Verification items for the finished model (mm, model axes). A direction names the side the tool comes from. Give positions to 0.01 mm unless a question says otherwise; leave off trailing zeros. Write each loop counter-clockwise with the first axis right and the second up, starting at its lowest first coordinate (ties: lowest second). Pieces come first, ordered by that corner, then holes. Notation, with made-up numbers: (-25, 69) - (-4, 69) arc R29 cw to (-4, 103) - close; hole circle Ø8 at (4, -33). An arc over 180 degrees is marked (long way). Put each result on its own line as item: value.
from build123d import *

# Parameters (mm, degrees)
SKETCH1_W           = 32
SKETCH1_H           = 32
SKETCH1_W_2         = 28
SKETCH1_H_2         = 28
BOSS_EXTRUDE1_DEPTH = 20
SKETCH2_W           = 10
SKETCH2_H           = 8
CUT_EXTRUDE1_DEPTH  = 33


with BuildPart() as part:
    # Sketch1 → Boss-Extrude1 (new body)
    with BuildSketch(Plane(origin=(0, 0, 0), x_dir=(1, 0, 0), z_dir=(0, 1, 0))):
        Rectangle(SKETCH1_W, SKETCH1_H)
        Rectangle(SKETCH1_W_2, SKETCH1_H_2, mode=Mode.SUBTRACT)
    extrude(amount=BOSS_EXTRUDE1_DEPTH)

    # Sketch2 → Cut-Extrude1 (cut, through all)
    with BuildSketch(Plane(origin=(16, 0, 0), x_dir=(0, 0, -1), z_dir=(1, 0, 0))):
        with Locations((0, 4)):
            Rectangle(SKETCH2_W, SKETCH2_H)
    extrude(amount=-CUT_EXTRUDE1_DEPTH, mode=Mode.SUBTRACT)


solid = part.part
Q1. Set-up check for faces 5 (the face through (0, 0, 15)), 6 (the face through (-14, 10, 0)), 7 (the face through (-15, 4, 5)): record each of +Z, -Z, +X, -X, +Y, -Y from which the full face is reachable in a straight line by a thin tool's end or side.
Answers follow:
face 5: +Z, -Z, +X, -X, -Y
face 6: +Y, -Y
face 7: +X, -X, -Y
Q2. Scan line: line 1 along Z through (x, y) = (0, 18.75). Record every from-to range of solid material in increasing order.
Answers follow:
line 1: z = -16 to -14, 14 to 16
Q3. Release check for a two-part mould opening along Z. For faces 1 (the face through (0, 10, -16)), 2 (the face through (-15, 4, -5)), 3 (the face through (16, 10, 0)), 4 (the face through (15, 4, 5)) record: released by +Z, released by -Z, zero draft, split by the parting line, or undercut.
Answers follow:
face 1: released by -Z
face 2: undercut
face 3: zero draft
face 4: undercut
Q4. Section check B-B, the plane x = 1. Record the cut outline in (y, z).
Answers follow:
outline: (0, -16) - (20, -16) - (20, -14) - (0, -14) - close; (0, 14) - (20, 14) - (20, 16) - (0, 16) - close
Q5. Section check A-A, the plane z = 3. Record the cut outline in (x, y), plus the area to 3 significant figures.
Answers follow:
outline: (-16, 8) - (-14, 8) - (-14, 20) - (-16, 20) - close; (14, 8) - (16, 8) - (16, 20) - (14, 20) - close
area: 48.0 mm2
Q6. Section check D-D, the plane y = 7.25. Record the cut outline in (x, z), plus the area to 3 significant figures.
Answers follow:
outline: (-16, -16) - (16, -16) - (16, -5) - (14, -5) - (14, -14) - (-14, -14) - (-14, -5) - (-16, -5) - close; (-16, 5) - (-14, 5) - (-14, 14) - (14, 14) - (14, 5) - (16, 5) - (16, 16) - (-16, 16) - close
area: 200 mm2
Q7. Go/stop test with flat-tipped pins: pin 1 Ø6 at (y, z) = (2.5, 1.5) entering from -X; pin 2 Ø0.6 at (x, z) = (15, 2) entering from -Y. Record where each tip stops, or that it passes through.
Answers follow:
pin 1: passes through
pin 2: stops at y = 8
Q8. Section check C-C, the plane y = 18. Record the cut outline in (x, z).
Answers follow:
outline: (-16, -16) - (16, -16) - (16, 16) - (-16, 16) - close; hole (-14, -14) - (14, -14) - (14, 14) - (-14, 14) - close
